from build123d import *

# Parameters (mm, degrees)
BOSS_EXTRUDE1_DEPTH = 90
SKETCH2_R           = 15
SKETCH2_R_2         = 3
CUT_EXTRUDE1_DEPTH  = 2
CUT_EXTRUDE2_DEPTH  = 2


with BuildPart() as part:
    # Sketch1 → Boss-Extrude1 (new body)
    with BuildSketch(Plane.XY):
        Polygon((0, 0), (0, 70), (49.497474683, 119.497474683), (129.497474683, 119.497474683), (129.497474683, 117.497474683), (49.497474683, 117.497474683), (2, 70), (2, 0), align=None)
    extrude(amount=BOSS_EXTRUDE1_DEPTH)

    # Sketch2 → Cut-Extrude1 (cut)
    with BuildSketch(Plane(origin=(0, 119.497474683, 0), x_dir=(1, 0, 0), z_dir=(0, 1, 0))):
        with Locations(Location((89.497474683, -45, 0), (0, 0, 270))):
            Circle(SKETCH2_R)
        with Locations(Location((59.497474683, -45, 0), (0, 0, 270))):
            Circle(SKETCH2_R_2)
        with Locations(Location((119.497474683, -10, 0), (0, 0, 270))):
            Circle(SKETCH2_R_2)
        with Locations(Location((119.497474683, -80, 0), (0, 0, 270))):
            Circle(SKETCH2_R_2)
    extrude(amount=-CUT_EXTRUDE1_DEPTH, mode=Mode.SUBTRACT)

    # Sketch3 → Cut-Extrude2 (cut)
    with BuildSketch(Plane.ZY):
        with BuildLine():
            Line((12, 60), (32, 60))
            ThreePointArc((32, 60), (37, 55), (32, 50))
            Line((32, 50), (12, 50))
            ThreePointArc((12, 50), (7, 55), (12, 60))
        make_face()
        with BuildLine():
            Line((58, 20), (78, 20))
            ThreePointArc((78, 20), (83, 15), (78, 10))
            Line((78, 10), (58, 10))
            ThreePointArc((58, 10), (53, 15), (58, 20))
        make_face()
        with BuildLine():
            Line((58, 60), (78, 60))
            ThreePointArc((78, 60), (83, 55), (78, 50))
            Line((78, 50), (58, 50))
            ThreePointArc((58, 50), (53, 55), (58, 60))
        make_face()
        with BuildLine():
            Line((12, 20), (32, 20))
            ThreePointArc((32, 20), (37, 15), (32, 10))
            Line((32, 10), (12, 10))
            ThreePointArc((12, 10), (7, 15), (12, 20))
        make_face()
    extrude(amount=-CUT_EXTRUDE2_DEPTH, mode=Mode.SUBTRACT)


solid = part.part
The model under review builds one solid part; all positions refer to its coordinate system, in mm. A direction names the side the tool comes from. Round coordinates to 2 decimals unless told otherwise and drop trailing zeros. Loops run counter-clockwise (first coordinate to the right, second up) from the corner with the lowest first, then second, coordinate; pieces in that order, holes last. Notation, with made-up numbers: (32, -12.75) -> (81, -12.75) arc R7 cw to (81, -7.75) -> close; hole circle Ø7 at (74.5, 64.25). An arc over 180 degrees is marked (long way). Return JSON: item names as keys, results as strings.
(1) Add section C-C on z = 10. Write out the cut boundary in (x, y), plus the area to 3 significant figures.
Solved:
{"outline": "(0, 0) -> (2, 0) -> (2, 10.42) -> (0, 10.42) -> close; (0, 19.58) -> (2, 19.58) -> (2, 50.42) -> (0, 50.42) -> close; (0, 59.58) -> (2, 59.58) -> (2, 70) -> (49.5, 117.5) -> (116.5, 117.5) -> (116.5, 119.5) -> (49.5, 119.5) -> (0, 70) -> close; (122.5, 117.5) -> (129.5, 117.5) -> (129.5, 119.5) -> (122.5, 119.5) -> close", "area": "348 mm2"}
(2) Add section B-B on y = 15. Write out the cut boundary in (x, z), plus the area to 3 significant figures.
Solved:
{"outline": "(0, 0) -> (2, 0) -> (2, 7) -> (0, 7) -> close; (0, 37) -> (2, 37) -> (2, 53) -> (0, 53) -> close; (0, 83) -> (2, 83) -> (2, 90) -> (0, 90) -> close", "area": "60.0 mm2"}
(3) Add section D-D on x = 80.5. Write out the cut boundary in (y, z).
Solved:
{"outline": "(117.5, 0) -> (119.5, 0) -> (119.5, 33) -> (117.5, 33) -> close; (117.5, 57) -> (119.5, 57) -> (119.5, 90) -> (117.5, 90) -> close"}
(4) The part is to be moulded in two halves that separate along Z. For faces 1 (the flat face through (70, 118, 90)), 2 (the flat face through (2, 35, 44)), 3 (the cylindrical face through (62.47, 118.51, 44.61)), 4 (the cylindrical face through (1, 15, 53)), say which applies: released by +Z, released by -Z, zero draft, split by the parting line, or undercut.
Solved:
{"face 1": "released by +Z", "face 2": "zero draft", "face 3": "undercut", "face 4": "undercut"}
(5) For pin 1 (2 mm diameter, centred on x = 1, z = 23.5, fed in from +Y); pin 2 (1.5 mm diameter, centred on x = 25, z = 39, fed in from +Y); pin 3 (5 mm diameter, centred on x = 119.5, z = 10, fed in from +Y); pin 4 (1.6 mm diameter, centred on x = 0.5, z = 69, fed in from +Y), all flat-tipped, find the tip position at first contact; note any pin that passes through.
Solved:
{"pin 1": "y = 72", "pin 2": "y = 95.75", "pin 3": "through", "pin 4": "y = 71.3"}
(6) Add section A-A on z = 45. Write out the cut boundary in (x, y).
Solved:
{"outline": "(0, 0) -> (2, 0) -> (2, 70) -> (49.5, 117.5) -> (56.5, 117.5) -> (56.5, 119.5) -> (49.5, 119.5) -> (0, 70) -> close; (62.5, 117.5) -> (74.5, 117.5) -> (74.5, 119.5) -> (62.5, 119.5) -> close; (104.5, 117.5) -> (129.5, 117.5) -> (129.5, 119.5) -> (104.5, 119.5) -> close"}
(7) For line 1 (X direction, y = 118, z = 10); line 2 (Y direction, x = 59, z = 6.5); line 3 (X direction, y = 54.5, z = 4.5), list the stretches that pass through material, from the lowest coordinate up.
Solved:
{"line 1": "48 to 116.5, 122.5 to 129.5", "line 2": "117.5 to 119.5", "line 3": "0 to 2"}
(8) For faces 5 (the cylindrical face through (116.57, 118.51, 9.35)), 6 (the flat face through (108, 117.497, 44)), 7 (the cylindrical face through (1, 55, 37)), list the 3-axis set-ups (+Z, -Z, +X, -X, +Y, -Y) from which the entire face can be reached by the end or side of a thin tool; tool diameter is ignored.
Solved:
{"face 5": "+Y, -Y", "face 6": "+Z, -Z, +X, -Y", "face 7": "+X, -X"}
